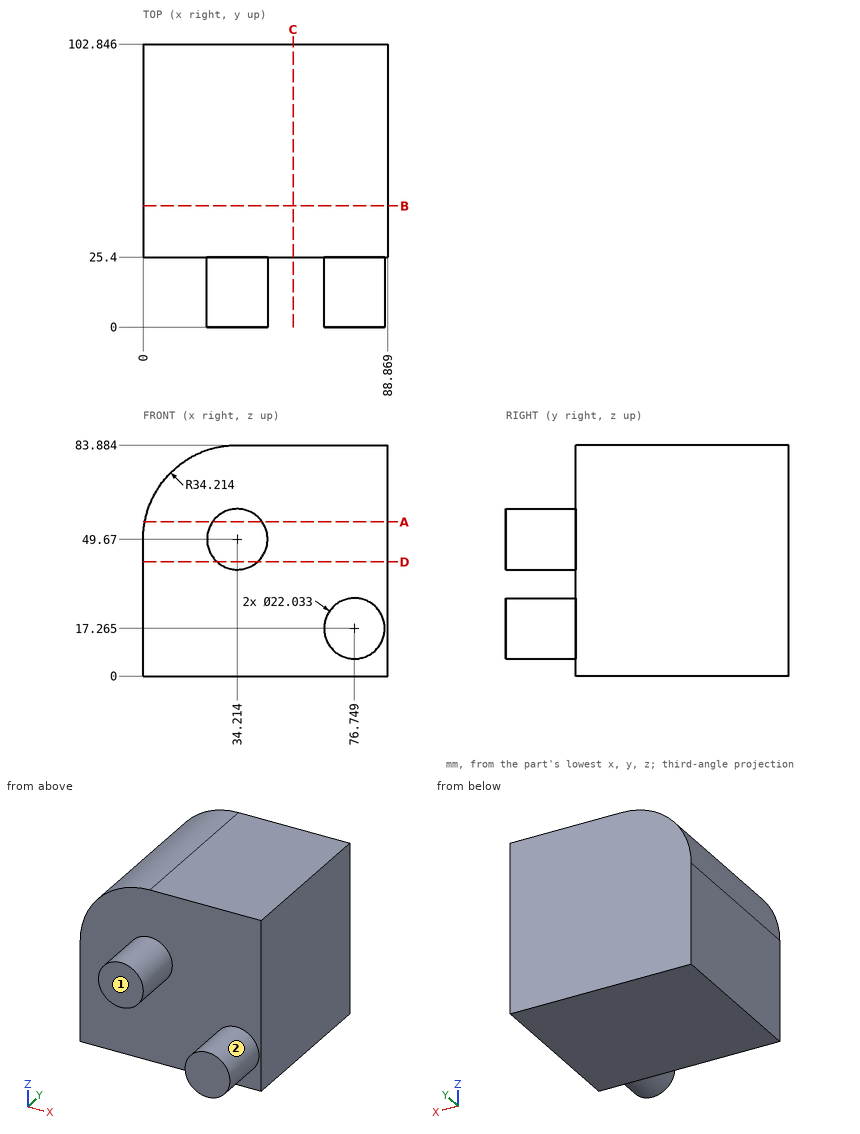
Can you work these out from the drawing? Everything is in mm from the part's minimum corner. A direction names the side the tool comes from. Round coordinates to 2 decimals unless told otherwise and drop trailing zeros. Loops run counter-clockwise (first coordinate to the right, second up) from the corner with the lowest first, then second, coordinate; pieces in that order, holes last. Notation, with made-up numbers: (84.5, 2) - (110.5, 2) arc R17 ccw to (110.5, 27) - close; hole circle Ø10 at (-22.75, 66). An arc over 180 degrees is marked (long way). Write item = value, one per line. Start each with the question number.
(1) If we section it at A-A (z = 56): Please give me the cut outline in (x, y).
(2) If we section it at C-C (x = 54.5): Please give me the cut outline in (y, z) (1 decimal).
(3) For the marked faces 1 and 2, which set-ups out of +Z, -Z, +X, -X, +Y, -Y let a thin tool reach every point of the face, with its end or its side?
(4) For P1, Ø4, axis at x = 43, z = 43, coming from the -Y side; P2, Ø1.5, axis at y = 83, z = 59.5, coming from the -X side; P3, Ø1.5, axis at x = 39, z = 22, coming from the -Y side, each with a flat end and sliding along its axis, tell me the tip position at first contact or that it passes through.
(5) If I drill on probe 1 along Z at (x, y) = (76.5, 21); probe 2 along Y at (x, z) = (39, 76); probe 3 along X at (y, z) = (82.5, 50.5), over which ranges is the centre line in solid material (lowest first)? Write a range as [from, to].
(6) If we section it at D-D (z = 41.5): Please give me the cut outline in (x, y) (1 decimal).
(7) If we section it at B-B (y = 44): Please give me the cut outline in (x, z) (1 decimal).
Ans:
q1.outline = (0.59, 25.4) - (25.2, 25.4) - (25.2, 0) - (43.23, 0) - (43.23, 25.4) - (88.87, 25.4) - (88.87, 102.85) - (0.59, 102.85) - close
q2.outline = (25.4, 0) - (102.8, 0) - (102.8, 83.9) - (25.4, 83.9) - close
q3.face_1 = +Z, -Z, +X, -X, -Y
q3.face_2 = -Y
q4.P1 = 0
q4.P2 = 1.23
q4.P3 = 25.4
q5.probe_1 = [6.25, 28.28]
q5.probe_2 = [25.4, 102.85]
q5.probe_3 = [0.01, 88.87]
q6.outline = (0, 25.4) - (26.8, 25.4) - (26.8, 0) - (41.6, 0) - (41.6, 25.4) - (88.9, 25.4) - (88.9, 102.8) - (0, 102.8) - close
q7.outline = (0, 0) - (88.9, 0) - (88.9, 83.9) - (34.2, 83.9) arc R34.2 ccw to (0, 49.7) - close
